The model under review builds one solid part; all positions refer to its coordinate system, in mm. A direction names the side the tool comes from. Round coordinates to 2 decimals unless told otherwise and drop trailing zeros. Order: outer loops, then holes, each group sorted by start corner. A loop starts at its lowest first (then second) coordinate and runs counter-clockwise, first axis right, second up. Notation, with made-up numbers: (21, -12) -> (54, -12) arc R24 cw to (54, 18) -> close; hole circle Ø5 at (-14, 39). An arc over 180 degrees is marked (long way). Return JSON: item names as keys, results as strings. Group by question number.
from build123d import *

# Parameters (mm, degrees)
SKETCH1_W           = 60
SKETCH1_H           = 19
BOSS_EXTRUDE1_DEPTH = 5
SKETCH2_W           = 60
SKETCH2_H           = 3
BOSS_EXTRUDE2_DEPTH = 20
BOSS_EXTRUDE3_DEPTH = 5
SKETCH4_R           = 1.67292172
CUT_EXTRUDE1_DEPTH  = 5
SKETCH5_R           = 2
CUT_EXTRUDE2_DEPTH  = 5


with BuildPart() as part:
    # Sketch1 → Boss-Extrude1 (new body)
    with BuildSketch(Plane.XY):
        with Locations((30, -9.5)):
            Rectangle(SKETCH1_W, SKETCH1_H)
    extrude(amount=BOSS_EXTRUDE1_DEPTH)

    # Sketch2 → Boss-Extrude2 (add)
    with BuildSketch(Plane.XY.offset(5)):
        with Locations((30, -17.5)):
            Rectangle(SKETCH2_W, SKETCH2_H)
    extrude(amount=BOSS_EXTRUDE2_DEPTH)

    # Sketch3 → Boss-Extrude3 (add)
    with BuildSketch(Plane(origin=(60, 0, 0), x_dir=(0, 0, -1), z_dir=(1, 0, 0))):
        Polygon((-5, 0), (-25, -16), (-5, -16), align=None)
    boss_extrude3 = extrude(amount=-BOSS_EXTRUDE3_DEPTH)

    # Mirror1: Boss-Extrude3 across plane
    add(boss_extrude3.mirror(Plane(origin=(30, 0, 0), x_dir=(0, 0, 1), z_dir=(1, 0, 0))))

    # Sketch4 → Cut-Extrude1 (cut)
    with BuildSketch(Plane.XY.offset(5)):
        with Locations((11, -8)):
            Circle(SKETCH4_R)
        with Locations((30, -8)):
            Circle(SKETCH4_R)
        with Locations((49, -8)):
            Circle(SKETCH4_R)
    extrude(amount=-CUT_EXTRUDE1_DEPTH, mode=Mode.SUBTRACT)

    # Sketch5 → Cut-Extrude2 (cut)
    with BuildSketch(Plane(origin=(0, -16, 0), x_dir=(1, 0, 0), z_dir=(0, 1, 0))):
        with Locations(Location((10, -15, 0), (0, 0, 270))):
            Circle(SKETCH5_R)
        with Locations(Location((30, -15, 0), (0, 0, 270))):
            Circle(SKETCH5_R)
        with Locations(Location((50, -15, 0), (0, 0, 270))):
            Circle(SKETCH5_R)
    extrude(amount=-CUT_EXTRUDE2_DEPTH, mode=Mode.SUBTRACT)


solid = part.part
Item 1: Consider section A-A on x = 30. State the section outline as (y, z) points, plus the area to 3 significant figures.
Item 2: Consider section C-C on y = -8. State the section outline as (x, z) points.
Item 3: Consider section D-D on z = 11.75. State the section outline as (x, y) points.
Item 4: Consider section B-B on z = 15. State the section outline as (x, y) points.
Item 5: Wall thickness on line 1 along X through (y, z) = (-1, 6); line 2 along X through (y, z) = (-17.5, 15); line 3 along Y through (x, z) = (11, 1.1): over which ranges is each line inside the solid? List them lowest first.
Item 6: Insertion check: pin 1 Ø6 at (x, z) = (27, 18) entering from +Y; pin 2 Ø3 at (x, y) = (30, -8) entering from -Z; pin 3 Ø4 at (x, y) = (49, -8) entering from +Z. Each pin has a flat end and moves straight along its axis. Give the tip position at first contact, or say it passes through.
Item 7: For faces 4 (the face through (30, -19, 12)), 5 (the face through (55, -11, 11)), list the 3-axis set-ups (+Z, -Z, +X, -X, +Y, -Y) from which the entire face can be reached by the end or side of a thin tool; tool diameter is ignored.
Item 8: The part is to be moulded in two halves that separate along X. For faces 1 (the face through (30, 0, 2)), 2 (the face through (0, -11, 10)), 3 (the face through (30, -6, 5)), say which applies: +X half, -X half, draft (parallel to the pull), parting line (faces both ways), or undercut.
Values:
{
 "1": {"outline": "(-19, 0) -> (-9.67, 0) -> (-9.67, 5) -> (-16, 5) -> (-16, 13) -> (-19, 13) -> close; (-19, 17) -> (-16, 17) -> (-16, 25) -> (-19, 25) -> close; (-6.33, 0) -> (0, 0) -> (0, 5) -> (-6.33, 5) -> close", "area": "126 mm^2"},
 "2": {"outline": "(0, 0) -> (9.33, 0) -> (9.33, 5) -> (5, 5) -> (5, 15) -> (0, 15) -> close; (12.67, 0) -> (28.33, 0) -> (28.33, 5) -> (12.67, 5) -> close; (31.67, 0) -> (47.33, 0) -> (47.33, 5) -> (31.67, 5) -> close; (50.67, 0) -> (60, 0) -> (60, 15) -> (55, 15) -> (55, 5) -> (50.67, 5) -> close"},
 "3": {"outline": "(0, -19) -> (60, -19) -> (60, -5.4) -> (55, -5.4) -> (55, -16) -> (5, -16) -> (5, -5.4) -> (0, -5.4) -> close"},
 "4": {"outline": "(0, -19) -> (8, -19) -> (8, -16) -> (5, -16) -> (5, -8) -> (0, -8) -> close; (12, -19) -> (28, -19) -> (28, -16) -> (12, -16) -> close; (32, -19) -> (48, -19) -> (48, -16) -> (32, -16) -> close; (52, -19) -> (60, -19) -> (60, -8) -> (55, -8) -> (55, -16) -> (52, -16) -> close"},
 "5": {"line 1": "0 to 5, 55 to 60", "line 2": "0 to 8, 12 to 28, 32 to 48, 52 to 60", "line 3": "-19 to -9.67, -6.33 to 0"},
 "6": {"pin 1": "y = -16", "pin 2": "through", "pin 3": "z = 5"},
 "7": {"face 4": "+Z, -Z, +X, -X, -Y", "face 5": "+Z, +Y"},
 "8": {"face 1": "draft", "face 2": "-X half", "face 3": "undercut"}
}
